Design review of the part shown in the three views and the two pictorial views. Dimensions are in mm from the part's minimum x, y and z. A direction names the side the tool comes from. Coordinates: 2 decimals unless noted, no trailing zeros. Loops run counter-clockwise (first coordinate to the right, second up) from the corner with the lowest first, then second, coordinate; pieces in that order, holes last. Notation, with made-up numbers: (0.5, -33.75) -> (5.5, -33.75) arc R11 ccw to (5.5, -22.75) -> close; hole circle Ø2 at (19, -14). An arc over 180 degrees is marked (long way). Use CSV: the item, a comma, the result in double quotes.
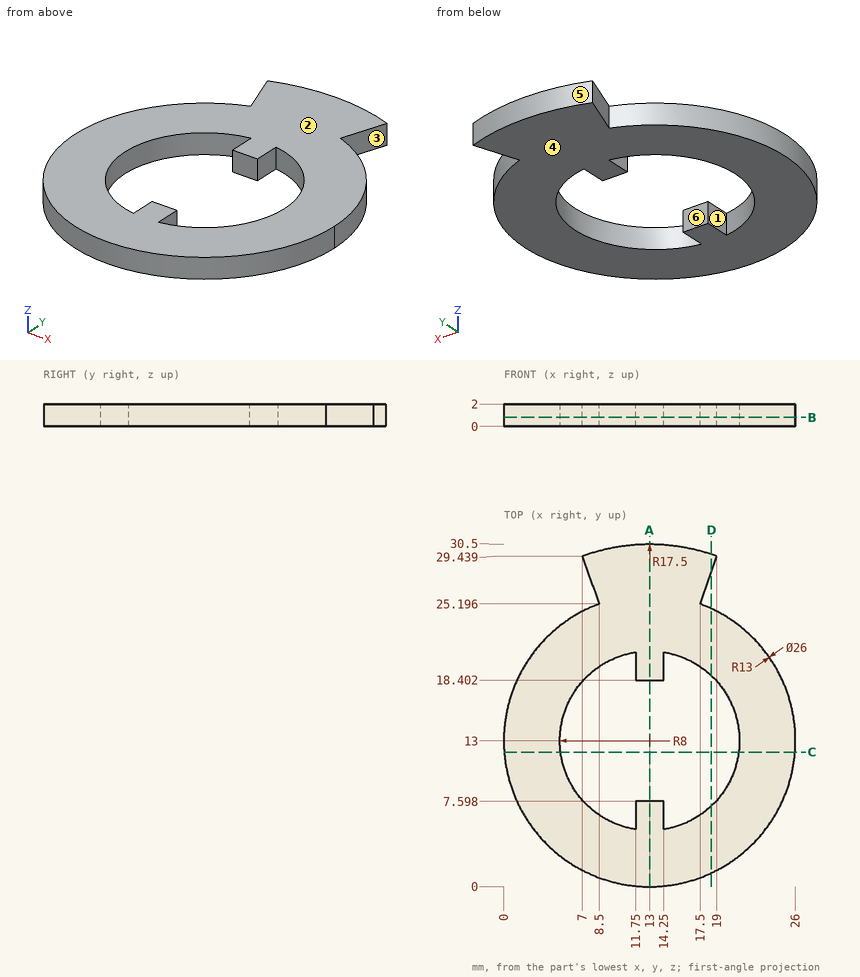
Item 1: To check wall thickness, follow line 1 along Y through (x, z) = (12.5, 0.95); line 2 along Y through (x, z) = (10, 1.9); line 3 along X through (y, z) = (16, 0.3). State the ranges of each line that lie inside material, in increasing order.
Checked values:
line 1,"0.01 to 7.6, 18.4 to 30.49"
line 2,"0.35 to 5.58, 20.42 to 30.24"
line 3,"0.35 to 5.58, 20.42 to 25.65"
Item 2: Add section B-B (z = 0.8). Give the boundary of the cut face in (x, y).
Checked values:
outline,"(7, 29.44) -> (8.5, 25.2) arc R13 ccw (long way) to (17.5, 25.2) -> (19, 29.44) arc R17.5 ccw to start; hole (11.75, 5.1) -> (11.75, 7.6) -> (14.25, 7.6) -> (14.25, 5.1) arc R8 ccw to (14.25, 20.9) -> (14.25, 18.4) -> (11.75, 18.4) -> (11.75, 20.9) arc R8 ccw to start"
Item 3: Add section D-D (x = 18.5). Give the boundary of the cut face in (y, z) (1 decimal).
Checked values:
outline,"(1.2, 0) -> (7.2, 0) -> (7.2, 2) -> (1.2, 2) -> close; (18.8, 0) -> (24.8, 0) -> (24.8, 2) -> (18.8, 2) -> close; (28, 0) -> (29.6, 0) -> (29.6, 2) -> (28, 2) -> close"
Item 4: Clearance check with flat-ended pins moving along their axes: pin 1 (0.6 mm diameter, centred on y = 19.5, z = 1, fed in from +X); pin 2 (0.6 mm diameter, centred on y = 6.5, z = 1, fed in from -X). State where each tip first meets the part, or that it passes through.
Checked values:
pin 1,"x = 24.43"
pin 2,"x = 1.57"
Item 5: Machinability: for the marked faces 1, 2 and 3, which of the approach directions +Z, -Z, +X, -X, +Y, -Y give a long, thin tool a straight path to every point of the face, cutting with its end or side? Answer none if there is none.
Checked values:
face 1,"+Z, -Z"
face 2,"+Z, +X, -X, +Y, -Y"
face 3,"+Z, -Z, +X"
Item 6: Add section C-C (y = 12). Give the boundary of the cut face in (x, z), then the cut area to 3 significant figures.
Checked values:
outline,"(0.04, 0) -> (5.06, 0) -> (5.06, 2) -> (0.04, 2) -> close; (20.94, 0) -> (25.96, 0) -> (25.96, 2) -> (20.94, 2) -> close"
area,"20.1 mm^2"
Item 7: Add section A-A (x = 13). Give the boundary of the cut face in (y, z).
Checked values:
outline,"(0, 0) -> (7.6, 0) -> (7.6, 2) -> (0, 2) -> close; (18.4, 0) -> (30.5, 0) -> (30.5, 2) -> (18.4, 2) -> close"
Item 8: Draft analysis for pull direction Y (two halves, no side actions). For the marked faces 4, 5 and 6, state which applies: pulls with the +Y half, pulls with the -Y half, needs draft (parallel to the pull), parting line crosses it, or undercut.
Checked values:
face 4,"needs draft"
face 5,"pulls with the +Y half"
face 6,"undercut"
